from build123d import *

# Parameters (mm, degrees)
SKETCH1_W           = 47
SKETCH1_H           = 14
SKETCH2_R           = 1.5
BOSS_EXTRUDE1_DEPTH = 15
CUT_EXTRUDE1_DEPTH  = 11.4


with BuildPart() as part:
    # Sketch1 → Revolve1 (revolve)
    with BuildSketch(Plane.XY):
        with Locations((23.5, 7)):
            Rectangle(SKETCH1_W, SKETCH1_H)
    revolve(axis=Axis((0, 0, 0), (1, 0, 0)))

    # Sketch2 → Boss-Extrude1 (add)
    with BuildSketch(Plane(origin=(47, 0, 0), x_dir=(0, 0, -1), z_dir=(1, 0, 0))):
        Circle(SKETCH2_R)
    extrude(amount=BOSS_EXTRUDE1_DEPTH)

    # Sketch3 → Cut-Extrude1 (cut)
    with BuildSketch(Plane(origin=(62, 0, 0), x_dir=(0, 0, -1), z_dir=(1, 0, 0))):
        with BuildLine():
            Line((-1.2, 0.9), (1.2, 0.9))
            ThreePointArc((1.2, 0.9), (0, 1.5), (-1.2, 0.9))
        make_face()
    extrude(amount=-CUT_EXTRUDE1_DEPTH, mode=Mode.SUBTRACT)


solid = part.part
Geometry: final body of the model. Coordinates: model frame, mm. A direction names the side the tool comes from. Give positions to 0.01 mm unless a question says otherwise; leave off trailing zeros. Write each loop counter-clockwise with the first axis right and the second up, starting at its lowest first coordinate (ties: lowest second). Pieces come first, ordered by that corner, then holes. Notation, with made-up numbers: (26.25, -35.5) - (53.25, -35.5) arc R23 cw to (53.25, -10.5) - close; hole circle Ø9 at (-8.5, -6). An arc over 180 degrees is marked (long way). Return JSON: item names as keys, results as strings. Group by question number.
1) Section C-C on x = 53. Return the cut outline in (y, z), plus the area to 3 significant figures.
2) Section D-D on x = 30.5. Return the cut outline in (y, z).
3) Section A-A on y = 0. Return the cut outline in (x, z), plus the area to 3 significant figures.
4) Line query: line 1 (X direction, y = 2, z = -1.5); line 2 (Y direction, x = 46, z = -0.5). Output: solid intervals per line, ascending.
5) Section B-B on z = 0. Return the cut outline in (x, y).
6) Set-up query: faces 1 (the cylindrical face through (54.395, -1.464, 0.325)), 2 (the flat face through (56, 0.9, 0)), 3 (the flat face through (0, 0, 0)). Return all of +Z, -Z, +X, -X, +Y, -Y with unobstructed straight access to the full face (end or side cutting, diameter ignored); none if empty.
7) First-contact query: P1, Ø1.2, axis at x = 54.5, z = 0.5, coming from the +Y side; P2, Ø8.5, axis at y = 2, z = -3.5, coming from the +X side; P3, Ø3, axis at x = 15.5, z = 10, coming from the -Y side; P4, Ø5, axis at x = 10.5, z = -5.5, coming from the -Y side. Flat tips, straight axial feed; report the tip coordinate or a pass-through.
Filled in:
{
 "1": {"outline": "(0.9, -1.2) - (0.9, 1.2) arc R1.5 ccw (long way) to start", "area": "6.06 mm^2"},
 "2": {"outline": "circle Ø28 at (0, 0)"},
 "3": {"outline": "(0, -14) - (47, -14) - (47, -1.5) - (62, -1.5) - (62, 1.5) - (47, 1.5) - (47, 14) - (0, 14) - close", "area": "1,360 mm^2"},
 "4": {"line 1": "x = 0 to 47", "line 2": "y = -13.99 to 13.99"},
 "5": {"outline": "(0, -14) - (47, -14) - (47, -1.5) - (62, -1.5) - (62, 0.9) - (50.6, 0.9) - (50.6, 1.5) - (47, 1.5) - (47, 14) - (0, 14) - close"},
 "6": {"face 1": "+X", "face 2": "+Z, -Z, +X, +Y", "face 3": "+Z, -Z, -X, +Y, -Y"},
 "7": {"P1": "stops at y = 0.9", "P2": "stops at x = 62", "P3": "stops at y = -11.12", "P4": "stops at y = -13.67"}
}
